Check sheet for the modelled part. Datum: model origin and axes. Units: mm. A direction names the side the tool comes from. Round coordinates to 2 decimals unless told otherwise and drop trailing zeros. Order: outer loops, then holes, each group sorted by start corner. A loop starts at its lowest first (then second) coordinate and runs counter-clockwise, first axis right, second up.
from build123d import *

# Parameters (mm, degrees)
ESQUISSE1_W        = 50
ESQUISSE1_H        = 20
ESQUISSE1_R        = 1.6
BOSS_EXTRU_1_DEPTH = 5
ESQUISSE2_W        = 26
ESQUISSE2_H        = 10
ESQUISSE2_R        = 1.5
BOSS_EXTRU_2_DEPTH = 20


with BuildPart() as part:
    # Esquisse1 → Boss.-Extru.1 (new body)
    with BuildSketch(Plane.XY):
        Rectangle(ESQUISSE1_W, ESQUISSE1_H)
        with Locations((-18.5, 0)):
            Circle(ESQUISSE1_R, mode=Mode.SUBTRACT)
        with Locations((18.5, 0)):
            Circle(ESQUISSE1_R, mode=Mode.SUBTRACT)
    extrude(amount=BOSS_EXTRU_1_DEPTH)

    # Esquisse2 → Boss.-Extru.2 (add)
    with BuildSketch(Plane(origin=(0, 10, 0), x_dir=(1, 0, 0), z_dir=(0, 1, 0))):
        Polygon((25, 0), (25, -5), (45, -39.641016151), (47.165063509, -38.391016151), align=None)
        Polygon((-45, -39.641016151), (-47.165063509, -38.391016151), (-25, 0), (-25, -5), align=None)
        with Locations((0, 5)):
            Rectangle(ESQUISSE2_W, ESQUISSE2_H)
        with Locations((-9, 5)):
            Circle(ESQUISSE2_R, mode=Mode.SUBTRACT)
        with Locations((9, 5)):
            Circle(ESQUISSE2_R, mode=Mode.SUBTRACT)
    extrude(amount=-BOSS_EXTRU_2_DEPTH)


solid = part.part
1) Sectioned sample at A-A on x = 18.5. Record the cut outline in (y, z).
2) Draft check along Z on faces 6 (the face through (-20.4, 0.1, 0)), 7 (the face through (7.8, 0.1, -4.1)), 8 (the face through (13, 0, -5)). Enter one of: pulls with the +Z half, pulls with the -Z half, needs draft (parallel to the pull), parting line crosses it, or undercut.
3) Gauge pin test, flat ends, axial feed: pin 1 (2 mm diameter, centred on x = 32.5, y = 4, fed in from -Z); pin 2 (1.5 mm diameter, centred on x = -28.5, y = -5.5, fed in from +Z); pin 3 (8 mm diameter, centred on y = 3.5, z = -6.5, fed in from +X). Record the tip position at first contact, or that the pin passes through.
4) Sectioned sample at C-C on y = 7. Record the cut outline in (x, z), and give its area (3 significant figures).
5) Scan lines: line 1 (X direction, y = 1.25, z = -5); line 2 (Z direction, x = 9, y = -5.25); line 3 (Z direction, x = -18, y = -6.75). Record each from-to range of solid material in increasing order.
6) Set-up check for faces 1 (the face through (20.25, 0.14, 0)), 2 (the face through (46.067, 0.14, 39.025)), 3 (the face through (0, 0, -10)), 4 (the face through (-13, 0, -5)), 5 (the face through (-34.86, 0.14, 22.08)): record each of +Z, -Z, +X, -X, +Y, -Y from which the full face is reachable in a straight line by a thin tool's end or side.
7) Sectioned sample at B-B on z = -5. Record the cut outline in (x, y), and give its area (3 significant figures).
8) Sectioned sample at D-D on z = 28. Record the cut outline in (x, y), and give its area (3 significant figures).
Values found:
1. outline: (-10, 0) - (-1.6, 0) - (-1.6, 5) - (-10, 5) - close; (1.6, 0) - (10, 0) - (10, 5) - (1.6, 5) - close
2. face 6: pulls with the -Z half
2. face 7: undercut
2. face 8: needs draft
3. pin 1: stops at z = 11.26
3. pin 2: stops at z = 12.36
3. pin 3: stops at x = 13
4. outline: (-47.17, 38.39) - (-25, 0) - (-13, 0) - (-13, -10) - (13, -10) - (13, 0) - (25, 0) - (47.17, 38.39) - (45, 39.64) - (25, 5) - (-25, 5) - (-45, 39.64) - close; hole circle Ø3 at (-9, -5); hole circle Ø3 at (9, -5)
4. area: 707 mm2
5. line 1: x = -13 to -10.5, -7.5 to 7.5, 10.5 to 13
5. line 2: z = -10 to -6.5, -3.5 to 5
5. line 3: z = 0 to 5
6. face 1: -Z, +X, +Y, -Y
6. face 2: +Z, +X, +Y, -Y
6. face 3: -Z, +X, -X, +Y, -Y
6. face 4: -Z, -X, +Y, -Y
6. face 5: +Z, +Y, -Y
7. outline: (-13, -10) - (-10.5, -10) - (-10.5, 10) - (-13, 10) - close; (-7.5, -10) - (7.5, -10) - (7.5, 10) - (-7.5, 10) - close; (10.5, -10) - (13, -10) - (13, 10) - (10.5, 10) - close
7. area: 400 mm2
8. outline: (-41.17, -10) - (-38.28, -10) - (-38.28, 10) - (-41.17, 10) - close; (38.28, -10) - (41.17, -10) - (41.17, 10) - (38.28, 10) - close
8. area: 115 mm2
